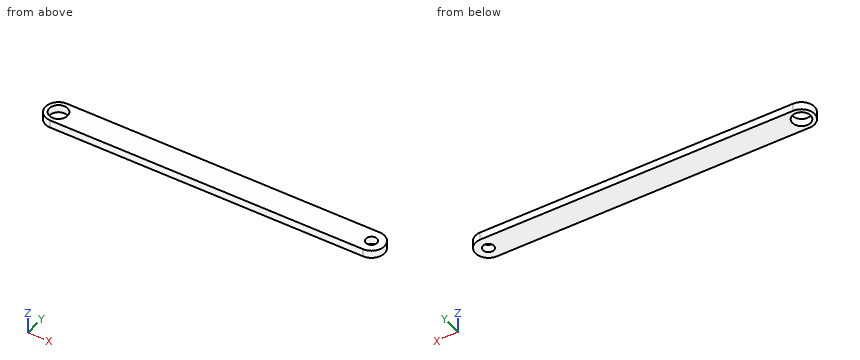
Autodesk Inventor part; units mm, degrees
ref_plane "YZ Plane" through (0, 0, 0) normal (1, 0, 0) x (0, 1, 0)
ref_plane "XZ Plane" through (0, 0, 0) normal (0, 1, 0) x (-1, 0, 0)
ref_plane "XY Plane" through (0, 0, 0) normal (0, 0, 1) x (1, 0, 0)
sketch "草圖1" plane through (0, 0, 0) normal (0, 0, 1) x (1, 0, 0)
  line L0 (-120, 0) -> (0, 0) construction
  line L1 (-120, -5) -> (0, -5)
  line L2 (0, 5) -> (-120, 5)
  arc A0 (-120, 5) -> (-120, -5) centre (-120, 0) ccw
  arc A1 (0, -5) -> (0, 5) centre (0, 0) ccw
  circle A2 centre (-120, 0) radius 3.5
  circle A3 centre (0, 0) radius 2.1
  point P0 (-60, 0)
  dimension "d0" = 120
  dimension "d1" = 10
  dimension "d2" = 7
  dimension "d3" = 4.2
extrude "擠出1" add sketch "草圖1" along normal blind 3
sketch "草圖4" plane through (0, 0, 3) normal (0, 0, 1) x (1, 0, 0)
  line L0 (2.932, 0.7895) -> (0.36, 2.1968)
  arc A0 (0.36, 2.1968) -> (-0.36, 2.1968) centre (0, 1.5389) ccw
  line L1 (-0.36, 2.1968) -> (-2.932, 0.7895)
  arc A1 (-2.932, 0.7895) -> (-2.932, -0.7895) centre (-2.5, 0) ccw
  line L2 (-2.932, -0.7895) -> (-0.36, -2.1968)
  arc A2 (-0.36, -2.1968) -> (0.36, -2.1968) centre (0, -1.5389) ccw
  line L3 (0.36, -2.1968) -> (2.932, -0.7895)
  arc A3 (2.932, -0.7895) -> (2.932, 0.7895) centre (2.5, 0) ccw
  circle A4 centre (0, 0) radius 1.55
extrude "擠出3" [suppressed]
properties part number "adjustable_120"
Work out the finished part from the listing and answer in its coordinate system (mm). Coordinates: 2 decimals unless noted, no trailing zeros. Loops run counter-clockwise (first coordinate to the right, second up) from the corner with the lowest first, then second, coordinate; pieces in that order, holes last. Notation, with made-up numbers: (57.5, -5.5) -> (75.5, -5.5) arc R36 cw to (75.5, 33.5) -> close; hole circle Ø10 at (-18, 44.25). An arc over 180 degrees is marked (long way). Write each question's results on one line, items separated by ' | '. Start each with the question number.
1) Find section B-B on z = 1.6. Determine the outline of the cut face in (x, y), then the cut area to 3 significant figures.
2) Consider line 1 along Y through (x, z) = (0, 0.8); line 2 along X through (y, z) = (-0.25, 2.05); line 3 along Y through (x, z) = (-120, 1.55). Determine where each line is inside the solid, lowest interval first.
3) Flat-ended cylindrical pins translate along their axes: P1, Ø6, axis at x = -19, y = 3.5, coming from the -Z side; P2, Ø4, axis at x = -120, y = 0, coming from the +Z side. Find the tip coordinate at first contact, or state that the pin passes through.
4) Find section A-A on y = 0. Determine the outline of the cut face in (x, z), then the cut area to 3 significant figures.
Response values:
1) outline: (-120, -5) -> (0, -5) arc R5 ccw to (0, 5) -> (-120, 5) arc R5 ccw to start; hole circle Ø7 at (-120, 0); hole circle Ø4.2 at (0, 0) | area: 1,230 mm^2
2) line 1: y = -5 to -2.1, 2.1 to 5 | line 2: x = -124.99 to -123.49, -116.51 to -2.09, 2.09 to 4.99 | line 3: y = -5 to -3.5, 3.5 to 5
3) P1: stops at z = 0 | P2: passes through
4) outline: (-125, 0) -> (-123.5, 0) -> (-123.5, 3) -> (-125, 3) -> close; (-116.5, 0) -> (-2.1, 0) -> (-2.1, 3) -> (-116.5, 3) -> close; (2.1, 0) -> (5, 0) -> (5, 3) -> (2.1, 3) -> close | area: 356 mm^2
